The model under review builds one solid part; all positions refer to its coordinate system, in mm. A direction names the side the tool comes from. Give positions to 0.01 mm unless a question says otherwise; leave off trailing zeros. Write each loop counter-clockwise with the first axis right and the second up, starting at its lowest first coordinate (ties: lowest second). Pieces come first, ordered by that corner, then holes. Notation, with made-up numbers: (-16.5, 3.5) - (24.5, 3.5) arc R11 ccw to (24.5, 24.5) - close; hole circle Ø2 at (60.5, 54.25). An arc over 180 degrees is marked (long way). Write item = value, one per line.
```python
from build123d import *

# Parameters (mm, degrees)
F0_W          = 8
F0_H          = 10
F1_DEPTH      = 15
F1_DEPTH_BACK = 15
F2_R          = 1
F3_DEPTH      = 30.001
F5_DEPTH      = 30.001
F6_R          = 1.2
F7_DEPTH      = 8.001


with BuildPart() as f1:
    # F0 (on Front) → F1 (new body, two sides)
    with BuildSketch(Plane.XZ) as f1_sk:
        Rectangle(F0_W, F0_H)
    extrude(amount=F1_DEPTH)
    extrude(f1_sk.sketch, amount=-F1_DEPTH_BACK)

    # F2 (on face) → F3 (cut, through all)
    with BuildSketch(Plane.XZ.offset(15)):
        with Locations((0, 2.5)):
            Circle(F2_R)
    extrude(amount=-F3_DEPTH, mode=Mode.SUBTRACT)

    # F4 (on face) → F5 (cut, through all)
    with BuildSketch(Plane.XZ.offset(15)):
        with BuildLine():
            Line((-2, 0), (-2, -5))
            Line((-2, -5), (2, -5))
            Line((2, -5), (2, 0))
            ThreePointArc((2, 0), (1.853553, 0.353553), (1.5, 0.5))
            Line((1.5, 0.5), (-1.5, 0.5))
            ThreePointArc((-1.5, 0.5), (-1.853553, 0.353553), (-2, 0))
        make_face()
    extrude(amount=-F5_DEPTH, mode=Mode.SUBTRACT)

    # F6 (on face) → F7 (cut, through all)
    with BuildSketch(Plane.YZ.offset(4)):
        with Locations((-9, -2)):
            Circle(F6_R)
        with Locations((9, -2)):
            Circle(F6_R)
    extrude(amount=-F7_DEPTH, mode=Mode.SUBTRACT)


solid = f1.part
```
1. For line 1 (Z direction, x = 3.2, y = 9); line 2 (X direction, y = -1.5, z = 0); line 3 (Z direction, x = 0, y = -12.5), list the stretches that pass through material, from the lowest coordinate up. Write a range as from..to.
Findings below:
line_1 = -5..-3.2, -0.8..5
line_2 = -4..-2, 2..4
line_3 = 0.5..1.5, 3.5..5
2. Take a section at B-B on y = 5.5. Give the boundary of the cut face in (x, z).
Findings below:
outline = (-4, -5) - (-2, -5) - (-2, 0) arc R0.5 cw to (-1.5, 0.5) - (1.5, 0.5) arc R0.5 cw to (2, 0) - (2, -5) - (4, -5) - (4, 5) - (-4, 5) - close; hole circle Ø2 at (0, 2.5)
3. Take a section at C-C on x = -3. Give the boundary of the cut face in (y, z), and give its area (3 significant figures).
Findings below:
outline = (-15, -5) - (15, -5) - (15, 5) - (-15, 5) - close; hole circle Ø2.4 at (-9, -2); hole circle Ø2.4 at (9, -2)
area = 291 mm²
4. Machinability: for faces 1 (the flat face through (2, 0, -3)), 2 (the flat face through (0, -15, 1)), which of the approach directions +Z, -Z, +X, -X, +Y, -Y give a long, thin tool a straight path to every point of the face, cutting with its end or side? Answer none if there is none.
Findings below:
face_1 = -Z, +Y, -Y
face_2 = +Z, -Z, +X, -X, -Y
5. Take a section at D-D on z = -2. Give the boundary of the cut face in (x, y).
Findings below:
outline = (-4, -15) - (-2, -15) - (-2, -10.2) - (-4, -10.2) - close; (-4, -7.8) - (-2, -7.8) - (-2, 7.8) - (-4, 7.8) - close; (-4, 10.2) - (-2, 10.2) - (-2, 15) - (-4, 15) - close; (2, -15) - (4, -15) - (4, -10.2) - (2, -10.2) - close; (2, -7.8) - (4, -7.8) - (4, 7.8) - (2, 7.8) - close; (2, 10.2) - (4, 10.2) - (4, 15) - (2, 15) - close
6. Take a section at A-A on z = 2.5. Give the boundary of the cut face in (x, y), and give its area (3 significant figures).
Findings below:
outline = (-4, -15) - (-1, -15) - (-1, 15) - (-4, 15) - close; (1, -15) - (4, -15) - (4, 15) - (1, 15) - close
area = 180 mm²
7. Draft analysis for pull direction X (two halves, no side actions). For faces 3 (the flat face through (0, 0, 5)), 4 (the flat face through (0, 0, 0.5)), 5 (the flat face through (-4, 0, 0)), state which applies: +X half, -X half, draft (parallel to the pull), parting line (faces both ways), or undercut.
Findings below:
face_3 = draft
face_4 = undercut
face_5 = -X half
8. Insertion check: P1, Ø1.5, axis at x = 0, y = -8.5, coming from the -Z side; P2, Ø1.4, axis at y = 9, z = -2, coming from the +X side. Each pin has a flat end and moves straight along its axis. Give the tip position at first contact, or say it passes through.
Findings below:
P1 = 0.5
P2 = through
